from build123d import *

# Parameters (mm, degrees)
BASPROSKE_W        = 20
BASPROSKE_H        = 12.5
TOOTHCUT_DEPTH     = 57.678920244
TEETHCUTS_COUNT    = 27
SKETCH1_R          = 33
CUT_EXTRUDE1_DEPTH = 3
SKETCH2_R          = 33
CUT_EXTRUDE2_DEPTH = 3


with BuildPart() as part:
    # BasProSke → Base-Revolve (revolve)
    with BuildSketch(Plane(origin=(0, 0, 0), x_dir=(1, 0, 0), z_dir=(0, 1, 0)), mode=Mode.PRIVATE) as base_revolve_sk:
        with Locations((10, 31.25)):
            Rectangle(BASPROSKE_W, BASPROSKE_H)
    revolve(base_revolve_sk.sketch.rotate(Axis((-10, 0, 0), (1, 0, 0)), 180), axis=Axis((-10, 0, 0), (1, 0, 0)))

    # TooCutSke → ToothCut (cut, through all)
    with BuildSketch(Plane(origin=(0, 0, 0), x_dir=(0, 0, -1), z_dir=(1, 0, 0))):
        with BuildLine():
            ThreePointArc((2.416400206, 24.85742656), (1.592639823, 27.277654117), (0.32737703, 29.499183468))
            ThreePointArc((0.32737703, 29.499183468), (0, 29.501), (-0.32737703, 29.499183468))
            ThreePointArc((-0.32737703, 29.499183468), (-1.592639823, 27.277654117), (-2.416400206, 24.85742656))
            ThreePointArc((-2.416400206, 24.85742656), (0, 24.9746), (2.416400206, 24.85742656))
        make_face()
    toothcut = extrude(amount=TOOTHCUT_DEPTH, mode=Mode.SUBTRACT)

    # TeethCuts: ToothCut ×27 about axis
    teethcuts_axis = Axis((0, 0, 0), (1, 0, 0))
    for i in range(1, TEETHCUTS_COUNT):
        add(toothcut.rotate(teethcuts_axis, i * 360 / TEETHCUTS_COUNT), mode=Mode.SUBTRACT)

    # Sketch1 → Cut-Extrude1 (cut)
    with BuildSketch(Plane(origin=(20, 0, 0), x_dir=(0, 0, -1), z_dir=(1, 0, 0))):
        Circle(SKETCH1_R)
    extrude(amount=-CUT_EXTRUDE1_DEPTH, mode=Mode.SUBTRACT)

    # Sketch2 → Cut-Extrude2 (cut)
    with BuildSketch(Plane.ZY):
        with Locations(Location((0, 0, 0), (0, 0, 180))):
            Circle(SKETCH2_R)
    extrude(amount=-CUT_EXTRUDE2_DEPTH, mode=Mode.SUBTRACT)


solid = part.part
Could you check a few things on this model? Use its own coordinates, in mm. Give positions to 0.01 mm unless a question says otherwise; leave off trailing zeros. Loops run counter-clockwise (first coordinate to the right, second up) from the corner with the lowest first, then second, coordinate; pieces in that order, holes last. Notation, with made-up numbers: M -23.75,7.25 L -3.75,7.25 A15 ccw -3.75,29.25 Z; hole C 7,-40 d11. An arc over 180 degrees is marked long. Answer as a JSON object with one key per item and string values.
Q1. Suppose I cut it at A-A, the plane y = 0. List the corners of the cut face in (x, z) for me, plus the area to 3 significant figures.
Values found:
{"outline": "M 0,-37.5 L 20,-37.5 L 20,-33 L 17,-33 L 17,-27.33 L 3,-27.33 L 3,-33 L 0,-33 Z; M 0,33 L 3,33 L 3,27.33 L 17,27.33 L 17,33 L 20,33 L 20,37.5 L 0,37.5 Z", "area": "339 mm²"}
Q2. For P1, Ø10, axis at x = 9, y = 20.5, coming from the -Z side; P2, Ø1, axis at x = 6.5, z = 9, coming from the -Y side; P3, Ø1, axis at x = 11.5, z = 14, coming from the +Y side, each with a flat end and sliding along its axis, tell me the tip position at first contact or that it passes through.
Values found:
{"P1": "stops at z = -34.15", "P2": "stops at y = -36.52", "P3": "stops at y = 34.99"}
Q3. If I drill on probe 1 along Y at (x, z) = (1.05, 0); probe 2 along Z at (x, y) = (6, 25); probe 3 along Z at (x, y) = (13, 5.5) (3 decimals), over which ranges is the centre line in solid material (lowest first)? Write a range as [from, to].
Values found:
{"probe 1": "y = [-37.5, -33], [33, 37.5]", "probe 2": "z = [-27.95, -13.66], [-10.71, -8.01], [-3.51, -2.38], [2.38, 3.51], [8.01, 10.71], [13.66, 27.95]", "probe 3": "z = [-37.094, -28.875], [28.875, 37.094]"}
